from build123d import *

# Parameters (mm, degrees)
F1_DEPTH = 25.4
F4_DEPTH = 121.295029
F5_W     = 172.064931
F5_H     = 53.261429
F5_H_2   = 25.4
F2_DEPTH = 28.615158
F6_R     = 21.58089
F3_DEPTH = 28.615158


with BuildPart() as f1:
    # F0 (on Top) → F1 (new body)
    with BuildSketch(Plane.XY):
        with BuildLine():
            ThreePointArc((0.07735, 86.408892), (61.127679, 61.072985), (86.408927, 0))
            ThreePointArc((86.408927, 0), (64.999971, -56.934229), (11.381807, -85.656039))
            Line((11.381807, -85.656039), (229.284793, -85.656039))
            Line((229.284793, -85.656039), (229.284793, 86.408892))
            Line((229.284793, 86.408892), (0.07735, 86.408892))
        make_face()
        with BuildLine():
            Line((0.07735, 52.184075), (0.07735, 86.408892))
            ThreePointArc((0.07735, 86.408892), (-86.223044, -5.66475), (11.381807, -85.656039))
            Line((11.381807, -85.656039), (0.07735, -85.656039))
            Line((0.07735, -85.656039), (0.07735, -52.184075))
            ThreePointArc((0.07735, -52.184075), (-52.184132, 0), (0.07735, 52.184075))
        make_face()
        with BuildLine():
            ThreePointArc((11.381807, -85.656039), (64.999971, -56.934229), (86.408927, 0))
            ThreePointArc((86.408927, 0), (61.127679, 61.072985), (0.07735, 86.408892))
            Line((0.07735, 86.408892), (0.07735, 52.184075))
            ThreePointArc((0.07735, 52.184075), (36.927091, 36.872397), (52.184132, 0))
            ThreePointArc((52.184132, 0), (36.927091, -36.872397), (0.07735, -52.184075))
            Line((0.07735, -52.184075), (0.07735, -85.656039))
            Line((0.07735, -85.656039), (11.381807, -85.656039))
        make_face()
    extrude(amount=F1_DEPTH)

    # F0 (on Top) → F4 (join)
    with BuildSketch(Plane.XY):
        with BuildLine():
            ThreePointArc((11.381807, -85.656039), (64.999971, -56.934229), (86.408927, 0))
            ThreePointArc((86.408927, 0), (61.127679, 61.072985), (0.07735, 86.408892))
            Line((0.07735, 86.408892), (0.07735, 52.184075))
            ThreePointArc((0.07735, 52.184075), (36.927091, 36.872397), (52.184132, 0))
            ThreePointArc((52.184132, 0), (36.927091, -36.872397), (0.07735, -52.184075))
            Line((0.07735, -52.184075), (0.07735, -85.656039))
            Line((0.07735, -85.656039), (11.381807, -85.656039))
        make_face()
        with BuildLine():
            Line((0.07735, 52.184075), (0.07735, 86.408892))
            ThreePointArc((0.07735, 86.408892), (-86.223044, -5.66475), (11.381807, -85.656039))
            Line((11.381807, -85.656039), (0.07735, -85.656039))
            Line((0.07735, -85.656039), (0.07735, -52.184075))
            ThreePointArc((0.07735, -52.184075), (-52.184132, 0), (0.07735, 52.184075))
        make_face()
    extrude(amount=F4_DEPTH)

    # F5 (on face) → F2 (join)
    with BuildSketch(Plane.YZ.offset(229.284793)):
        with Locations((0.376427, -26.630714)):
            Rectangle(F5_W, F5_H)
        with Locations((0.376427, 12.7)):
            Rectangle(F5_W, F5_H_2)
    extrude(amount=-F2_DEPTH)

    # F6 (on face) → F3 (cut, through all)
    with BuildSketch(Plane.YZ.offset(229.284793)):
        with Locations((-47.304388, -26.372436)):
            Circle(F6_R)
        with Locations((48.057241, -26.372436)):
            Circle(F6_R)
    extrude(amount=-F3_DEPTH, mode=Mode.SUBTRACT)


solid = f1.part
Work out the finished part from the listing and answer in its coordinate system (mm). A direction names the side the tool comes from. Round coordinates to 2 decimals unless told otherwise and drop trailing zeros. Loops run counter-clockwise (first coordinate to the right, second up) from the corner with the lowest first, then second, coordinate; pieces in that order, holes last. Notation, with made-up numbers: (16, 86.5) -> (51, 86.5) arc R10 cw to (51, 95.5) -> close; hole circle Ø11 at (67, 30.25). An arc over 180 degrees is marked (long way). Use one line per item in the form item = value.
(1) For a pull along Y with two mould halves and no side action, classify faces 4 (the cylindrical face through (215.18, 68.64, -19.89)), 5 (the flat face through (215, -1, -53.261)), 6 (the cylindrical face through (215.18, -26.72, -19.89)), 7 (the flat face through (215, -85.656, -26)) as released by +Y, released by -Y, zero draft, split by the parting line, or undercut.
Answer list:
face_4 = undercut
face_5 = zero draft
face_6 = undercut
face_7 = released by -Y
(2) A tool of negligible diameter and unlimited length cuts with its end or side. For faces 1 (the flat face through (37.2, -37.2, 121.295)), 2 (the flat face through (200.67, -1, -22)), 3 (the flat face through (119, -85.656, 13)), from which of +Z, -Z, +X, -X, +Y, -Y can it reach the whole face along a straight path? Write none if from no direction.
Answer list:
face_1 = +Z, +X, -X, +Y, -Y
face_2 = -Z, -X, +Y, -Y
face_3 = +Z, -Z, +X, -Y
(3) Find section D-D on x = 191. Give the vertices of the cut face in (y, z).
Answer list:
outline = (-85.66, 0) -> (86.41, 0) -> (86.41, 25.4) -> (-85.66, 25.4) -> close
(4) Find section A-A on y = -41.5. Give the vertices of the cut face in (x, z), then the cut area to 3 significant figures.
Answer list:
outline = (-75.79, 0) -> (-31.64, 0) -> (-31.64, 121.3) -> (-75.79, 121.3) -> close; (31.64, 0) -> (200.67, 0) -> (200.67, -5.59) -> (229.28, -5.59) -> (229.28, 25.4) -> (75.79, 25.4) -> (75.79, 121.3) -> (31.64, 121.3) -> close; (200.67, -53.26) -> (229.28, -53.26) -> (229.28, -47.16) -> (200.67, -47.16) -> close
area = 14,900 mm2
(5) Find section B-B on z = 15.5. Give the vertices of the cut face in (x, y), then the cut area to 3 significant figures.
Answer list:
outline = (0.08, 86.41) arc R86.41 ccw (long way) to (11.38, -85.66) -> (229.28, -85.66) -> (229.28, 86.41) -> close; hole (0.08, -52.18) arc R52.18 ccw to (52.18, 0) arc R52.18 ccw to (0.08, 52.18) arc R52.18 ccw to start
area = 42,600 mm2
(6) Find section C-C on x = 8. Give the vertices of the cut face in (y, z), then the cut area to 3 significant figures.
Answer list:
outline = (-86.04, 0) -> (-51.57, 0) -> (-51.57, 121.3) -> (-86.04, 121.3) -> close; (51.57, 0) -> (86.41, 0) -> (86.41, 25.4) -> (86.04, 25.4) -> (86.04, 121.3) -> (51.57, 121.3) -> close
area = 8,370 mm2
(7) Straight lines are drawn through the part: line 1 (Z direction, x = 174, y = -67.5); line 2 (Z direction, x = -63.5, y = 50.5); line 3 (Y direction, x = 174.5, z = 17). For each, find the intervals that lie inside material, in ascending order.
Answer list:
line_1 = 0 to 25.4
line_2 = 0 to 121.3
line_3 = -85.66 to 86.41
(8) Flat-ended cylindrical pins translate along their axes: P1, Ø12, axis at y = 5.5, z = 95, coming from the -X side; P2, Ø10, axis at x = 88, y = -11, coming from the -Z side; P3, Ø1, axis at y = -26, z = 9, coming from the -X side; P4, Ø12, axis at x = 37, z = 51.5, coming from the +Y side. Find the tip coordinate at first contact, or state that the pin passes through.
Answer list:
P1 = -86.41
P2 = 0
P3 = -82.56
P4 = 80.66
